Can you work these out from the model? Positions are in its coordinate system, mm. A direction names the side the tool comes from. Give positions to 0.01 mm unless a question says otherwise; leave off trailing zeros. Loops run counter-clockwise (first coordinate to the right, second up) from the corner with the lowest first, then second, coordinate; pieces in that order, holes last. Notation, with made-up numbers: (11, 81.5) - (59, 81.5) arc R23 cw to (59, 100.5) - close; hole circle Ø7 at (35, 24). An arc over 180 degrees is marked (long way). Write item = value, one per line.
Autodesk Inventor part; units mm, degrees
ref_plane "YZ Plane" through (0, 0, 0) normal (1, 0, 0) x (0, 1, 0)
ref_plane "XZ Plane" through (0, 0, 0) normal (0, 1, 0) x (-1, 0, 0)
ref_plane "XY Plane" through (0, 0, 0) normal (0, 0, 1) x (1, 0, 0)
sketch "Sketch1" plane through (0, 0, 0) normal (0, 0, 1) x (1, 0, 0)
  circle A0 centre (0, 0) radius 79.375
  line L0 (82.2618, 32.9086) -> (107.6618, 32.9086)
  line L1 (107.6618, 32.9086) -> (107.6618, -0.1114)
  line L2 (-88.5728, 7.62) -> (-98.7328, 7.62)
  line L3 (-98.7328, 7.62) -> (-98.7328, 0)
  line L4 (0, 96.3985) -> (20.32, 96.3985)
  line L5 (20.32, 96.3985) -> (20.32, 86.2385)
  line L6 (82.2618, -32.9086) -> (107.6618, -32.9086)
  line L7 (107.6618, -32.9086) -> (107.6618, -0.1114)
  line L8 (-88.2741, -7.5943) -> (-98.7328, -7.5943)
  line L9 (-98.7328, -7.5943) -> (-98.7328, 0)
  line L10 (0, 96.3985) -> (-20.32, 96.3985)
  line L11 (-20.32, 96.3985) -> (-20.32, 86.5466)
  arc A1 (-88.2741, -7.5943) -> (-20.32, -86.2385) centre (0, 0) ccw
  arc A2 (-20.32, 86.5466) -> (-88.5728, 7.62) centre (0, 0) ccw
  arc A3 (20.32, -86.2385) -> (82.2618, -32.9086) centre (0, 0) ccw
  arc A4 (82.2618, 32.9086) -> (20.32, 86.2385) centre (0, 0) ccw
  line L12 (-88.9, 0) -> (88.9, 0) construction
  line L13 (0, -96.3985) -> (20.32, -96.3985)
  line L14 (20.32, -96.3985) -> (20.32, -86.2385)
  line L15 (0, -96.3985) -> (-20.32, -96.3985)
  line L16 (-20.32, -96.3985) -> (-20.32, -86.2385)
  arc A5 (-20.32, 86.5466) -> (-88.5728, 7.62) centre (0, 0) ccw
  arc A6 (82.2618, 32.9086) -> (20.32, 86.2385) centre (0, 0) ccw
  arc A7 (-88.2741, -7.5943) -> (-20.32, -86.2385) centre (0, 0) ccw
  arc A8 (20.32, -86.2385) -> (82.2618, -32.9086) centre (0, 0) ccw
  line L17 (0, 0) -> (0, 96.3985) construction
  line L18 (0, 0) -> (0, -96.3985) construction
  dimension "d2" = 25.4
  dimension "d5" = 10.16
  dimension "d7" = 10.16
  dimension "d8" = 7.62
  dimension "d10" = 33.02
  dimension "d14" = 158.75
  dimension "d15" = 177.8
  dimension "d24" = 20.32
  dimension "d25" = 20.32
  dimension "d26" = 40.64
extrude "Extrusion2" add sketch "Sketch1" along normal mid plane 25.4
properties part number "celestronTubeBracket" material "Aluminum 6061"
Q1. I need wall thicknesses on L1, parallel to Y at x = 0, z = 3.25 (1 decimal); L2, parallel to X at y = 87, z = 7.5; L3, parallel to X at y = 25, z = -9.5. Which ranges of each line are inside material? Lowest first, please.
Output:
L1 = -96.4 to -79.4, 79.4 to 96.4
L2 = -20.32 to 20.32
L3 = -85.31 to -75.34, 75.34 to 107.66
Q2. We'd pull the mould along Y, two halves only. Please class faces 1 (the cylindrical face through (75.71, -23.84, -0.18)), 2 (the flat face through (95, 32.909, 0)), 3 (the flat face through (107.662, 0, 0)), 4 (the flat face through (95, -32.909, 0)): released by +Y, released by -Y, zero draft, split by the parting line, or undercut.
Output:
face_1 = undercut
face_2 = released by +Y
face_3 = zero draft
face_4 = released by -Y
Q3. Imagine slicing it at C-C, the plane y = 0. Write out the boundary of the cut face in (x, z) (3 decimals).
Output:
outline = (-98.733, -12.7) - (-79.375, -12.7) - (-79.375, 12.7) - (-98.733, 12.7) - close; (79.375, -12.7) - (107.662, -12.7) - (107.662, 12.7) - (79.375, 12.7) - close
Q4. For pin 1 (12.5 mm diameter, centred on x = 98.5, z = -6, fed in from +Y); pin 2 (3 mm diameter, centred on y = 89, z = 5, fed in from -X); pin 3 (3 mm diameter, centred on x = -92, z = -4.5, fed in from +Y), each with a flat end and sliding along its axis, tell me the tip position at first contact or that it passes through.
Output:
pin_1 = 32.91
pin_2 = -20.32
pin_3 = 7.62
Q5. Imagine slicing it at B-B, the plane x = 0. Write out the boundary of the cut face in (y, z) (1 decimal), then the cut area to 3 significant figures.
Output:
outline = (-96.4, -12.7) - (-79.4, -12.7) - (-79.4, 12.7) - (-96.4, 12.7) - close; (79.4, -12.7) - (96.4, -12.7) - (96.4, 12.7) - (79.4, 12.7) - close
area = 865 mm2
Q6. Which directions (+Z, -Z, +X, -X, +Y, -Y) give clear straight access to the entire face, cutting with the end or side of a thin tool? Please do faces 5 (the flat face through (-20.32, -91, 0)), 6 (the flat face through (20.32, 91, 0)), 7 (the flat face through (20.32, -91, 0)), 8 (the flat face through (-20.32, 92, 0)).
Output:
face_5 = +Z, -Z, -X, -Y
face_6 = +Z, -Z, +X, +Y
face_7 = +Z, -Z, +X, -Y
face_8 = +Z, -Z, -X, +Y
